Check sheet for the modelled part. Datum: model origin and axes. Units: mm. Give positions to 0.01 mm unless a question says otherwise; leave off trailing zeros. Write each loop counter-clockwise with the first axis right and the second up, starting at its lowest first coordinate (ties: lowest second). Pieces come first, ordered by that corner, then holes. Notation, with made-up numbers: M 12.5,20.5 L 46.5,20.5 A9 cw 46.5,32.5 Z; hole C 37,-37.5 d10. An arc over 180 degrees is marked long. Write item = value, one per line. Start each with the question number.
1) Cross-section at A-A, the plane x = 95. Record the cut outline in (y, z).
2) Cross-section at C-C, the plane z = 3. Give the number of separate pieces and of enclosed holes in the cut face, plus the area to 3 significant figures.
3) Cross-section at D-D, the plane y = 59. Record the cut outline in (x, z), plus the area to 3 significant figures.
4) Scan lines: line 1 along Y through (x, z) = (45, 2.3); line 2 along X through (y, z) = (78, 1.85); line 3 along X through (y, z) = (21.5, 1.2). Record each from-to range of solid material in increasing order. Write a range as [from, to].
5) Cross-section at B-B, the plane y = 30. Record the cut outline in (x, z), plus the area to 3 significant figures.
6) Go/stop test with flat-tipped pins: pin 1 (1 mm diameter, centred on x = 13.5, z = 3.5, fed in from -Y); pin 2 (1.8 mm diameter, centred on y = 20, z = 2, fed in from -X); pin 3 (2.5 mm diameter, centred on x = 45, y = 78, fed in from -Z); pin 4 (3 mm diameter, centred on x = 28, z = 4.5, fed in from +Y). Record where each tip stops, or that it passes through.
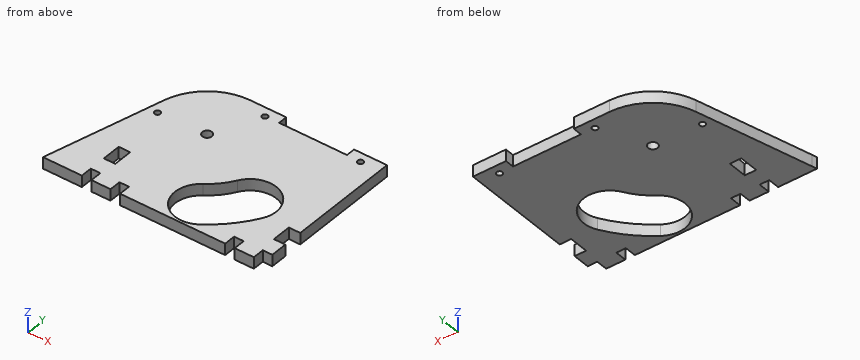
```python
from build123d import *

# Parameters (mm, degrees)
SKETCH1_R           = 2.5
BOSS_EXTRUDE1_DEPTH = 6
SKETCH2_W           = 5
SKETCH2_H           = 6
SKETCH2_W_2         = 6
SKETCH2_H_2         = 10
CUT_EXTRUDE1_DEPTH  = 134.97761007
SKETCH3_R           = 1.5
CUT_EXTRUDE2_DEPTH  = 134.97761007
SKETCH4_W           = 35.5
SKETCH4_H           = 4.75
CUT_EXTRUDE3_DEPTH  = 10
CAVITY1_OUTLINE_R   = 1.5
CAVITY1_DEPTH       = 6
CUT_EXTRUDE4_DEPTH  = 134.97761007


# Read off the part's stored shape, not the designer's step: Cavity1
with BuildPart() as part:
    # Sketch1 → Boss-Extrude1 (new body)
    with BuildSketch(Plane.XY):
        with BuildLine():
            Line((-9.685424338, 2.488484559), (5.386220056, 61.148792841))
            ThreePointArc((5.386220056, 61.148792841), (15.733633721, 76.897010412), (33.561388608, 83))
            Line((33.561388608, 83), (105, 83))
            Line((105, 83), (105, 0))
            Line((105, 0), (-10.324792855, 0))
            Line((-10.324792855, 0), (-9.685424338, 2.488484559))
        make_face()
        with Locations((33.561388608, 53.909722104)):
            Circle(SKETCH1_R, mode=Mode.SUBTRACT)
        with BuildLine():
            ThreePointArc((67.975974789, 4.760599446), (77.719162031, 13.288409394), (85.405906554, 23.707967867))
            ThreePointArc((85.405906554, 23.707967867), (80.896997447, 40.800941239), (63.804024076, 36.292032133))
            ThreePointArc((63.804024076, 36.292032133), (59.320089771, 30.213956356), (53.63656388, 25.239400554))
            ThreePointArc((53.63656388, 25.239400554), (50.566868781, 7.830294546), (67.975974789, 4.760599446))
        make_face(mode=Mode.SUBTRACT)
    extrude(amount=BOSS_EXTRUDE1_DEPTH)

    # Sketch2 → Cut-Extrude1 (cut, through all)
    with BuildSketch(Plane.XY.offset(6)):
        with Locations((12.5, 3)):
            Rectangle(SKETCH2_W, SKETCH2_H)
        with Locations((102.5, 3)):
            Rectangle(SKETCH2_W, SKETCH2_H)
        with Locations((27.5, 3)):
            Rectangle(SKETCH2_W, SKETCH2_H)
        with Locations((87.5, 3)):
            Rectangle(SKETCH2_W, SKETCH2_H)
        with Locations((102, 19.75)):
            Rectangle(SKETCH2_W_2, SKETCH2_H_2)
        with Locations((13, 19.75)):
            Rectangle(SKETCH2_W_2, SKETCH2_H_2)
    extrude(amount=-CUT_EXTRUDE1_DEPTH, mode=Mode.SUBTRACT)

    # Sketch3 → Cut-Extrude2 (cut, through all)
    with BuildSketch(Plane.XY.offset(6)):
        with Locations((95, 78)):
            Circle(SKETCH3_R)
        with Locations((45, 78)):
            Circle(SKETCH3_R)
    extrude(amount=-CUT_EXTRUDE2_DEPTH, mode=Mode.SUBTRACT)

    # Sketch4 → Cut-Extrude3 (cut)
    with BuildSketch(Plane.XY.offset(6)):
        with Locations((70, 80.625)):
            Rectangle(SKETCH4_W, SKETCH4_H)
    extrude(amount=-CUT_EXTRUDE3_DEPTH, mode=Mode.SUBTRACT)

    # Cavity1 outline → Cavity1 (cut)
    with BuildSketch(Plane.XY):
        with Locations((8.414860226, 52.844005614)):
            Circle(CAVITY1_OUTLINE_R)
    extrude(amount=CAVITY1_DEPTH, mode=Mode.SUBTRACT)

    # Sketch5 → Cut-Extrude4 (cut, through all)
    with BuildSketch(Plane.XY.offset(6)):
        with BuildLine():
            ThreePointArc((52.919593335, 26.263340609), (49.542928725, 7.113324), (68.692945334, 3.736659391))
            ThreePointArc((68.692945334, 3.736659391), (78.639115644, 12.442132046), (86.486000678, 23.078764654))
            ThreePointArc((86.486000678, 23.078764654), (81.526200661, 41.881035363), (62.723929952, 36.921235346))
            ThreePointArc((62.723929952, 36.921235346), (58.400136158, 31.060233704), (52.919593335, 26.263340609))
        make_face()
    extrude(amount=-CUT_EXTRUDE4_DEPTH, mode=Mode.SUBTRACT)


solid = part.part
```
Reply:
q1.outline = M 0,0 L 76.5,0 L 76.5,6 L 0,6 Z; M 79.5,0 L 83,0 L 83,6 L 79.5,6 Z
q2.separate_pieces = 1
q2.enclosed_holes = 6
q2.area = 6,980 mm2
q3.outline = M 4.83,0 L 105,0 L 105,6 L 4.83,6 Z
q3.area = 601 mm2
q4.line_1 = [0, 76.5], [79.5, 83]
q4.line_2 = [17.25, 43.5], [46.5, 93.5], [96.5, 105]
q4.line_3 = [-4.8, 10], [16, 48.69], [85.53, 99]
q5.outline = M -2.62,0 L 57.38,0 L 57.38,6 L -2.62,6 Z; M 88.35,0 L 105,0 L 105,6 L 88.35,6 Z
q5.area = 460 mm2
q6.pin_1 = 6
q6.pin_2 = -5.42
q6.pin_3 = through
q6.pin_4 = 82.72
